```python
from build123d import *

# Parameters (mm, degrees)
F0_W            = 192.8
F0_H            = 71.8
F0_W_2          = 188
F0_H_2          = 67
F1_DEPTH        = 35
F2_R            = 3
F3_DEPTH        = 192.801
F4_R            = 3.9
F5_DEPTH        = 25
F6_R            = 3
F7_DEPTH        = 25
F11_DEPTH       = 192.801
F12_DEPTH       = 71.801
F13_D           = 2.7
F13_DEPTH       = 12
F13_CSINK_D     = 5.5
F13_CSINK_ANGLE = 63
F13_TIP         = 0.8111618357
F15_D           = 2.7
F15_DEPTH       = 12
F15_CSINK_D     = 5.5
F15_CSINK_ANGLE = 63
F15_TIP         = 0.8111618357
F16_START       = -18.1
F16_DEPTH       = 112.3
F17_R           = 3
F18_DEPTH       = 25


with BuildPart() as f1:
    # F0 (on Top) → F1 (new body)
    with BuildSketch(Plane.XY):
        Rectangle(F0_W, F0_H)
        Rectangle(F0_W_2, F0_H_2, mode=Mode.SUBTRACT)
    extrude(amount=F1_DEPTH)

    # F2 (on face) → F3 (cut, through all)
    with BuildSketch(Plane(origin=(-96.4, 0, 0), x_dir=(0, -1, 0), z_dir=(-1, 0, 0))):
        with Locations((-17.95, 17.5)):
            Circle(F2_R)
        with Locations((17.95, 17.5)):
            Circle(F2_R)
    extrude(amount=-F3_DEPTH, mode=Mode.SUBTRACT)

    # F4 (on face) → F5 (cut)
    with BuildSketch(Plane.XZ.offset(35.9)):
        with Locations((0, 17.5)):
            Circle(F4_R)
        with Locations((33, 17.5)):
            Circle(F4_R)
        with Locations((66, 17.5)):
            Circle(F4_R)
        with Locations((-33, 17.5)):
            Circle(F4_R)
        with Locations((-66, 17.5)):
            Circle(F4_R)
    extrude(amount=-F5_DEPTH, mode=Mode.SUBTRACT)

    # F6 (on face) → F7 (cut)
    with BuildSketch(Plane(origin=(0, 35.9, 0), x_dir=(-1, 0, 0), z_dir=(0, 1, 0))):
        with Locations((0, 17.5)):
            Circle(F6_R)
        with Locations((33, 17.5)):
            Circle(F6_R)
        with Locations((66, 17.5)):
            Circle(F6_R)
        with Locations((-33, 17.5)):
            Circle(F6_R)
        with Locations((-66, 17.5)):
            Circle(F6_R)
    extrude(amount=-F7_DEPTH, mode=Mode.SUBTRACT)

    # F9 (on face) → F11 (cut, through all)
    with BuildSketch(Plane(origin=(-96.4, 0, 0), x_dir=(0, -1, 0), z_dir=(-1, 0, 0))):
        with BuildLine():
            Line((-7.6885714286, 26), (-24.5562429894, 26))
            Line((-24.5562429894, 26), (-20.95, 17.5))
            ThreePointArc((-20.95, 17.5), (-17.95, 20.5), (-14.95, 17.5))
            Line((-14.95, 17.5), (-7.6885714286, 26))
        make_face()
        Polygon((0, 35), (-28.3746179193, 35), (-24.5562429894, 26), (-7.6885714286, 26), align=None)
        Polygon((28.3215269446, 35), (0, 35), (7.6885714286, 26), (24.5304559445, 26), align=None)
        with BuildLine():
            Line((24.5304559445, 26), (7.6885714286, 26))
            Line((7.6885714286, 26), (14.95, 17.5))
            ThreePointArc((14.95, 17.5), (17.95, 20.5), (20.95, 17.5))
            Line((20.95, 17.5), (24.5304559445, 26))
        make_face()
        Polygon((7.6885714286, 26), (0, 35), (-7.6885714286, 26), align=None)
    extrude(amount=-F11_DEPTH, mode=Mode.SUBTRACT)

    # F10 (on face) → F12 (cut, through all)
    with BuildSketch(Plane.XZ.offset(35.9)):
        Polygon((-49.5, 35), (-82.5, 35), (-76.02, 26), (-55.98, 26), align=None)
        Polygon((-16.5, 35), (-49.5, 35), (-43.02, 26), (-22.98, 26), align=None)
        Polygon((-43.02, 26), (-49.5, 35), (-55.98, 26), align=None)
        Polygon((16.5, 35), (-16.5, 35), (-10.02, 26), (10.02, 26), align=None)
        Polygon((-10.02, 26), (-16.5, 35), (-22.98, 26), align=None)
        Polygon((49.5, 35), (16.5, 35), (22.98, 26), (43.02, 26), align=None)
        Polygon((55.98, 26), (49.5, 35), (43.02, 26), align=None)
        Polygon((82.5, 35), (49.5, 35), (55.98, 26), (76.02, 26), align=None)
        with BuildLine():
            ThreePointArc((69.9, 17.5), (66, 21.4), (62.1, 17.5))
            Line((62.1, 17.5), (69.9, 17.5))
        make_face()
        with BuildLine():
            ThreePointArc((36.9, 17.5), (33, 21.4), (29.1, 17.5))
            Line((29.1, 17.5), (36.9, 17.5))
        make_face()
        with BuildLine():
            ThreePointArc((3.9, 17.5), (0, 21.4), (-3.9, 17.5))
            Line((-3.9, 17.5), (3.9, 17.5))
        make_face()
        with BuildLine():
            ThreePointArc((-29.1, 17.5), (-33, 21.4), (-36.9, 17.5))
            Line((-36.9, 17.5), (-29.1, 17.5))
        make_face()
        with BuildLine():
            ThreePointArc((-62.1, 17.5), (-66, 21.4), (-69.9, 17.5))
            Line((-69.9, 17.5), (-62.1, 17.5))
        make_face()
        Polygon((22.98, 26), (16.5, 35), (10.02, 26), align=None)
    extrude(amount=-F12_DEPTH, mode=Mode.SUBTRACT)

    # F13
    with Locations(Plane.XZ.offset(35.9)):
        with Locations((-89, 30), (-89, 7.4), (89, 30), (89, 7.4)):
            CounterSinkHole(F13_D / 2, F13_CSINK_D / 2, depth=F13_DEPTH, counter_sink_angle=F13_CSINK_ANGLE)
            with Locations((0, 0, -(F13_DEPTH + F13_TIP / 2))):  # 118° drill point
                Cone(0, F13_D / 2, F13_TIP, mode=Mode.SUBTRACT)

    # F15
    with Locations(Plane(origin=(0, 35.9, 0), x_dir=(-1, 0, 0), z_dir=(0, 1, 0))):
        with Locations((89.0000388026, 30.0000663847), (89.0000388026, 7.4000651948), (-88.9999940991, 30.0000663847), (-88.9999940991, 7.4000651948)):
            CounterSinkHole(F15_D / 2, F15_CSINK_D / 2, depth=F15_DEPTH, counter_sink_angle=F15_CSINK_ANGLE)
            with Locations((0, 0, -(F15_DEPTH + F15_TIP / 2))):  # 118° drill point
                Cone(0, F15_D / 2, F15_TIP, mode=Mode.SUBTRACT)

    # F10 (on face) → F16 (cut)
    with BuildSketch(Plane.XZ.offset(35.9).offset(F16_START)):
        with BuildLine():
            Line((-55.98, 26), (-76.02, 26))
            Line((-76.02, 26), (-69.9, 17.5))
            ThreePointArc((-69.9, 17.5), (-66, 21.4), (-62.1, 17.5))
            Line((-62.1, 17.5), (-55.98, 26))
        make_face()
        with BuildLine():
            Line((-22.98, 26), (-43.02, 26))
            Line((-43.02, 26), (-36.9, 17.5))
            ThreePointArc((-36.9, 17.5), (-33, 21.4), (-29.1, 17.5))
            Line((-29.1, 17.5), (-22.98, 26))
        make_face()
        with BuildLine():
            Line((10.02, 26), (-10.02, 26))
            Line((-10.02, 26), (-3.9, 17.5))
            ThreePointArc((-3.9, 17.5), (0, 21.4), (3.9, 17.5))
            Line((3.9, 17.5), (10.02, 26))
        make_face()
        with BuildLine():
            Line((43.02, 26), (22.98, 26))
            Line((22.98, 26), (29.1, 17.5))
            ThreePointArc((29.1, 17.5), (33, 21.4), (36.9, 17.5))
            Line((36.9, 17.5), (43.02, 26))
        make_face()
        with BuildLine():
            Line((76.02, 26), (55.98, 26))
            Line((55.98, 26), (62.1, 17.5))
            ThreePointArc((62.1, 17.5), (66, 21.4), (69.9, 17.5))
            Line((69.9, 17.5), (76.02, 26))
        make_face()
    extrude(amount=-F16_DEPTH, mode=Mode.SUBTRACT)

    # F17 (on face) → F18 (cut)
    with BuildSketch(Plane(origin=(0, 35.9, 0), x_dir=(-1, 0, 0), z_dir=(0, 1, 0))):
        with Locations((0, 7.25)):
            Circle(F17_R)
    extrude(amount=-F18_DEPTH, mode=Mode.SUBTRACT)


solid = f1.part
```
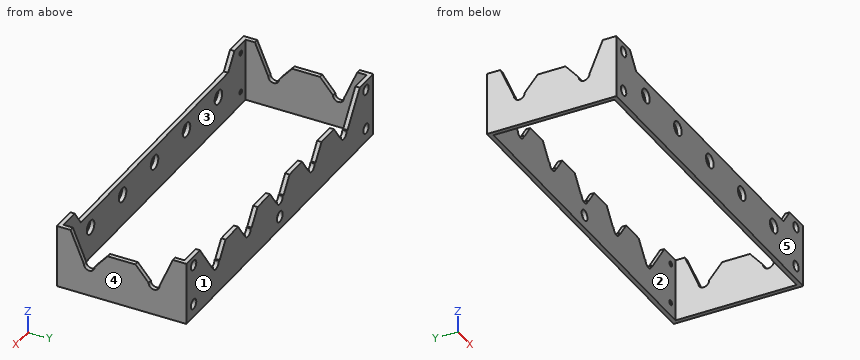
Input: part model. Units: mm. Frame: model coordinates. Face numbers are marked on the shaded views. A direction names the side the tool comes from. Give positions to 0.01 mm unless a question says otherwise; leave off trailing zeros. Order: outer loops, then holes, each group sorted by start corner. A loop starts at its lowest first (then second) coordinate and runs counter-clockwise, first axis right, second up. Notation, with made-up numbers: (38, 20.5) - (79, 20.5) arc R16 ccw to (79, 32.5) - close; hole circle Ø4 at (8, -9.5). An arc over 180 degrees is marked (long way). One line per item, written item: value.
1. Pin query (flat end, axial travel): pin 1 Ø5 at (x, z) = (0, 7.25) entering from +Y; pin 2 Ø1.2 at (x, y) = (-46.5, 35) entering from +Z; pin 3 Ø0.7 at (x, y) = (-69.5, 35) entering from +Z. Return the tip coordinate at first contact, or that it passes through.
Determined:
pin 1: y = -33.5
pin 2: z = 26
pin 3: z = 17.5
2. Cut plane C-C, the plane x = -66. Output: boundary loops of the cut face in (y, z).
Determined:
outline: (-35.9, 0) - (-33.5, 0) - (-33.5, 13.6) - (-35.9, 13.6) - close; (-35.9, 21.4) - (-33.5, 21.4) - (-33.5, 26) - (-35.9, 26) - close; (33.5, 0) - (35.9, 0) - (35.9, 14.5) - (33.5, 14.5) - close
3. Reachability of the marked faces 1 and 2 from +Z, -Z, +X, -X, +Y, -Y: full face, straight path, thin tool, end or side. Return the list, or none.
Determined:
face 1: +Z, -Z, +X, -X, +Y
face 2: +Z, -Z
4. Draft query along X for the marked faces 3, 4 and 5. Return one class per face: released by +X, released by -X, zero draft, split by the parting line, or undercut.
Determined:
face 3: undercut
face 4: released by +X
face 5: zero draft
5. Cut plane D-D, the plane y = -17.95. Output: boundary loops of the cut face in (x, z).
Determined:
outline: (-96.4, 0) - (-94, 0) - (-94, 14.5) - (-96.4, 14.5) - close; (94, 0) - (96.4, 0) - (96.4, 14.5) - (94, 14.5) - close
6. Cut plane A-A, the plane x = 0. Output: boundary loops of the cut face in (y, z).
Determined:
outline: (-35.9, 0) - (-33.5, 0) - (-33.5, 13.6) - (-35.9, 13.6) - close; (-35.9, 21.4) - (-33.5, 21.4) - (-33.5, 26) - (-35.9, 26) - close; (33.5, 0) - (35.9, 0) - (35.9, 4.25) - (33.5, 4.25) - close; (33.5, 10.25) - (35.9, 10.25) - (35.9, 14.5) - (33.5, 14.5) - close
7. Line query: probe 1 along Y at (x, z) = (-17.5, 9); probe 2 along Z at (x, y) = (0, 34); probe 3 along X at (y, z) = (-10.5, 18.5). Output: solid intervals per line, ascending.
Determined:
probe 1: -35.9 to -33.5, 33.5 to 35.9
probe 2: 0 to 4.25, 10.25 to 14.5
probe 3: -96.4 to -94, 94 to 96.4
8. Cut plane B-B, the plane y = 4.5. Output: boundary loops of the cut face in (x, z).
Determined:
outline: (-96.4, 0) - (-94, 0) - (-94, 26) - (-96.4, 26) - close; (94, 0) - (96.4, 0) - (96.4, 26) - (94, 26) - close
